Can you work these out from the drawing? Everything is in mm from the part's minimum corner. A direction names the side the tool comes from. Coordinates: 2 decimals unless noted, no trailing zeros. Loops run counter-clockwise (first coordinate to the right, second up) from the corner with the lowest first, then second, coordinate; pieces in that order, holes last.
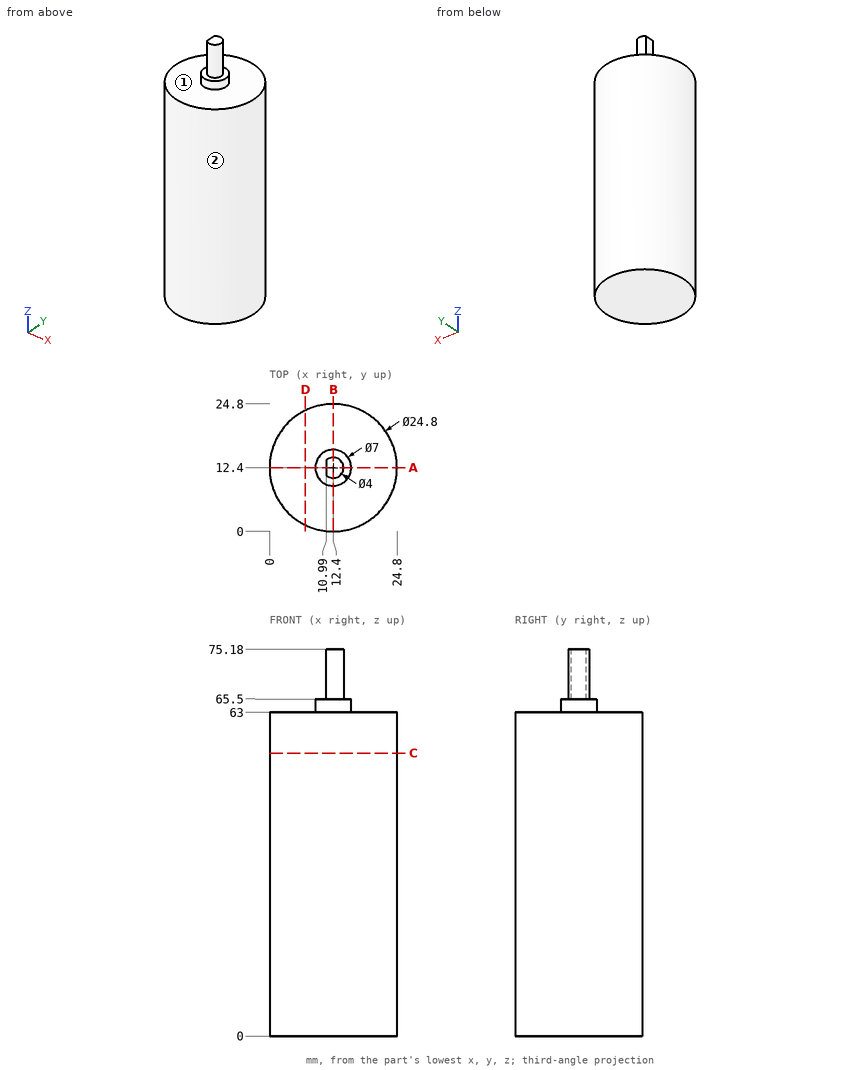
Item 1: On a 3-axis mill with a long thin cutter (end or side, diameter ignored), from which of +Z, -Z, +X, -X, +Y, -Y can I reach the whole of each face in a straight line? I mean the marked faces 1 and 2. Say none if no direction works.
Results are:
face 1: +Z
face 2: +Z, -Z
Item 2: Suppose I cut it at D-D, the plane x = 7. Please give me the cut outline in (y, z), plus the area to 3 significant figures.
Results are:
outline: (1.24, 0) - (23.56, 0) - (23.56, 63) - (1.24, 63) - close
area: 1,410 mm2
Item 3: Suppose I cut it at A-A, the plane y = 12.4. Please give me the cut outline in (x, z), plus the area to 3 significant figures.
Results are:
outline: (0, 0) - (24.8, 0) - (24.8, 63) - (15.9, 63) - (15.9, 65.5) - (14.4, 65.5) - (14.4, 75.18) - (10.99, 75.18) - (10.99, 65.5) - (8.9, 65.5) - (8.9, 63) - (0, 63) - close
area: 1,610 mm2
Item 4: I'm going to push flat-ended pins straight in: P1, Ø8, axis at y = 17.5, z = 31, coming from the -X side; P2, Ø2.5, axis at y = 12, z = 68, coming from the -X side; P3, Ø3, axis at x = 21.5, z = 27, coming from the -Y side. Where does each tip first touch, or does it pass through?
Results are:
P1: stops at x = 0.05
P2: stops at x = 10.99
P3: stops at y = 2.6
Item 5: Suppose I cut it at C-C, the plane z = 55. Please give me the cut outline in (x, y).
Results are:
outline: circle Ø24.8 at (12.4, 12.4)
Item 6: I need wall thicknesses on line 1 along X through (y, z) = (12.25, 34.5); line 2 along Z through (x, y) = (19, 4.25); line 3 along Z through (x, y) = (13.25, 9.25). Which ranges of each line are inside material? Lowest first, please.
Results are:
line 1: x = 0 to 24.8
line 2: z = 0 to 63
line 3: z = 0 to 65.5
Item 7: Suppose I cut it at B-B, the plane x = 12.4. Please give me the cut outline in (y, z).
Results are:
outline: (0, 0) - (24.8, 0) - (24.8, 63) - (15.9, 63) - (15.9, 65.5) - (14.4, 65.5) - (14.4, 75.18) - (10.4, 75.18) - (10.4, 65.5) - (8.9, 65.5) - (8.9, 63) - (0, 63) - close
